```python
from build123d import *

# Parameters (mm, degrees)
SKETCH1_W           = 145
SKETCH1_H           = 25
BOSS_EXTRUDE1_DEPTH = 10
SKETCH2_W           = 17.5
SKETCH2_H           = 32
BOSS_EXTRUDE2_DEPTH = 10
SKETCH4_W           = 73.5
SKETCH4_H           = 32
BOSS_EXTRUDE3_DEPTH = 10
SKETCH8_R           = 2.25
CUT_EXTRUDE5_DEPTH  = 193.888568868
SKETCH9_W           = 7.3
SKETCH9_H           = 4
CUT_EXTRUDE6_DEPTH  = 10
CUT_EXTRUDE7_REACH  = 195.92
SKETCH10_R          = 3.65
SKETCH11_R          = 12.75
CUT_EXTRUDE8_DEPTH  = 7
CUT_EXTRUDE11_REACH = 196.098
SKETCH14_R          = 1.65
CHAMFER1_SIZE       = 1.5
CHAMFER1_SIZE2      = 0.866025404
FILLET1_R           = 15
SKETCH15_R          = 2.25
CUT_EXTRUDE12_DEPTH = 195.692064553
CUT_EXTRUDE13_DEPTH = 4


with BuildPart() as part:
    # Sketch1 → Boss-Extrude1 (new body)
    with BuildSketch(Plane(origin=(0, 0, 0), x_dir=(1, 0, 0), z_dir=(0, 1, 0))):
        with Locations((72.5, 12.5)):
            Rectangle(SKETCH1_W, SKETCH1_H)
    extrude(amount=BOSS_EXTRUDE1_DEPTH)

    # Sketch2 → Boss-Extrude2 (add)
    with BuildSketch(Plane(origin=(0, 10, 0), x_dir=(1, 0, 0), z_dir=(0, 1, 0))):
        with Locations((153.75, 16)):
            Rectangle(SKETCH2_W, SKETCH2_H)
    extrude(amount=-BOSS_EXTRUDE2_DEPTH)

    # Sketch4 → Boss-Extrude3 (add)
    with BuildSketch(Plane.XZ):
        with Locations((154.25, -16)):
            Rectangle(SKETCH4_W, SKETCH4_H)
    extrude(amount=BOSS_EXTRUDE3_DEPTH)

    # Sketch8 → Cut-Extrude5 (cut, through all)
    with BuildSketch(Plane(origin=(0, 0, -25), x_dir=(-1, 0, 0), z_dir=(0, 0, -1))):
        with Locations((-137, 5)):
            Circle(SKETCH8_R)
        with Locations((-101, 5)):
            Circle(SKETCH8_R)
        with Locations(Location((-44, 5, 0), (0, 0, 180))):
            Circle(SKETCH8_R)
        with Locations(Location((-8, 5, 0), (0, 0, 180))):
            Circle(SKETCH8_R)
    extrude(amount=-CUT_EXTRUDE5_DEPTH, mode=Mode.SUBTRACT)

    # Sketch9 → Cut-Extrude6 (cut)
    with BuildSketch(Plane(origin=(0, 10, 0), x_dir=(1, 0, 0), z_dir=(0, 1, 0))):
        with Locations((137, 20)):
            Rectangle(SKETCH9_W, SKETCH9_H)
        with Locations((137, 5)):
            Rectangle(SKETCH9_W, SKETCH9_H)
        with Locations((101, 5)):
            Rectangle(SKETCH9_W, SKETCH9_H)
        with Locations((101, 20)):
            Rectangle(SKETCH9_W, SKETCH9_H)
        with Locations((8, 20)):
            Rectangle(SKETCH9_W, SKETCH9_H)
        with Locations((44, 20)):
            Rectangle(SKETCH9_W, SKETCH9_H)
        with Locations((44, 5)):
            Rectangle(SKETCH9_W, SKETCH9_H)
        with Locations((8, 5)):
            Rectangle(SKETCH9_W, SKETCH9_H)
    extrude(amount=-CUT_EXTRUDE6_DEPTH, mode=Mode.SUBTRACT)

    # Sketch10 → Cut-Extrude7 (cut, up to next)
    with BuildSketch(Plane(origin=(0, 0, 0), x_dir=(1, 0, 0), z_dir=(0, 1, 0)), mode=Mode.PRIVATE) as cut_extrude7_sk1:
        with Locations(Location((176, 16, 0), (0, 0, 270))):
            Circle(SKETCH10_R)
    cut_extrude7_tool1 = extrude(cut_extrude7_sk1.sketch, amount=-CUT_EXTRUDE7_REACH, mode=Mode.PRIVATE) & part.part
    add(cut_extrude7_tool1.solids().sort_by_distance((176, 0, -16))[0], mode=Mode.SUBTRACT)

    # Sketch11 → Cut-Extrude8 (cut)
    with BuildSketch(Plane.XZ.offset(10)):
        with Locations(Location((176, -16, 0), (0, 0, 270))):
            Circle(SKETCH11_R)
    extrude(amount=-CUT_EXTRUDE8_DEPTH, mode=Mode.SUBTRACT)

    # Sketch14 → Cut-Extrude11 (cut, up to next)
    with BuildSketch(Plane.XZ.offset(3), mode=Mode.PRIVATE) as cut_extrude11_sk1:
        with Locations(Location((176, -7.5, 0), (0, 0, 270))):
            Circle(SKETCH14_R)
    cut_extrude11_tool1 = extrude(cut_extrude11_sk1.sketch, amount=-CUT_EXTRUDE11_REACH, mode=Mode.PRIVATE) & part.part
    # Sketch14 → Cut-Extrude11 (cut, up to next)
    with BuildSketch(Plane.XZ.offset(3), mode=Mode.PRIVATE) as cut_extrude11_sk2:
        with Locations(Location((176, -24.5, 0), (0, 0, 270))):
            Circle(SKETCH14_R)
    cut_extrude11_tool2 = extrude(cut_extrude11_sk2.sketch, amount=-CUT_EXTRUDE11_REACH, mode=Mode.PRIVATE) & part.part
    add(cut_extrude11_tool1.solids().sort_by_distance((176, -3, -7.5))[0], mode=Mode.SUBTRACT)
    add(cut_extrude11_tool2.solids().sort_by_distance((176, -3, -24.5))[0], mode=Mode.SUBTRACT)

    # Chamfer1
    chamfer1_edges = [part.edges().sort_by_distance(p)[0] for p in [
        (176, 0, -5.85),
        (176, 0, -22.85),
    ]]
    chamfer1_side = [part.faces().sort_by_distance(p)[0] for p in [
        (162.928514877, 0, -16),
    ]]
    chamfer(chamfer1_edges, length=CHAMFER1_SIZE, length2=CHAMFER1_SIZE2, reference=chamfer1_side[0])

    # Fillet1
    fillet1_edges = [part.edges().sort_by_distance(p)[0] for p in [
        (162.5, 5, -32),
        (162.5, 5, 0),
        (191, -5, -32),
        (191, -5, 0),
    ]]
    fillet(fillet1_edges, radius=FILLET1_R)

    # Sketch15 → Cut-Extrude12 (cut, through all)
    with BuildSketch(Plane(origin=(0, 10, 0), x_dir=(1, 0, 0), z_dir=(0, 1, 0))):
        with Locations(Location((57.5, 12.5, 0), (0, 0, 270))):
            Circle(SKETCH15_R)
        with Locations(Location((87.5, 12.5, 0), (0, 0, 270))):
            Circle(SKETCH15_R)
    extrude(amount=-CUT_EXTRUDE12_DEPTH, mode=Mode.SUBTRACT)

    # Sketch16 → Cut-Extrude13 (cut)
    with BuildSketch(Plane(origin=(0, 10, 0), x_dir=(1, 0, 0), z_dir=(0, 1, 0))):
        Polygon((91.714656965, 12.5), (89.607328483, 16.15), (85.392671517, 16.15), (83.285343035, 12.5), (85.392671517, 8.85), (89.607328483, 8.85), align=None)
        Polygon((61.714656965, 12.5), (59.607328483, 16.15), (55.392671517, 16.15), (53.285343035, 12.5), (55.392671517, 8.85), (59.607328483, 8.85), align=None)
    extrude(amount=-CUT_EXTRUDE13_DEPTH, mode=Mode.SUBTRACT)


solid = part.part
```
Design review of the part built by this model. Coordinates are the model's own, in mm. A direction names the side the tool comes from. Coordinates: 2 decimals unless noted, no trailing zeros. Write each loop counter-clockwise with the first axis right and the second up, starting at its lowest first coordinate (ties: lowest second). Pieces come first, ordered by that corner, then holes.
1) Add section B-B (y = -8). Write out the cut boundary in (x, z), plus the area to 3 significant figures.
2) Add section C-C (x = 142.5). Write out the cut boundary in (y, z).
3) Add section D-D (x = 32). Write out the cut boundary in (y, z), plus the area to 3 significant figures.
4) Mouldability with a two-part tool opening along X and no side actions: class faces 4 (the flat face through (133.35, 5, -5)), 5 (the flat face through (131, 0, -28)), 6 (the flat face through (140.65, 5, -20)) as +X half, -X half, draft (parallel to the pull), parting line (faces both ways), or undercut.
5) Add section A-A (x = 87.5). Write out the cut boundary in (y, z).
6) To check wall thickness, follow L1, parallel to Z at x = 46, y = 7.5; L2, parallel to X at y = -1.75, z = -16.5; L3, parallel to Y at x = 137, z = -15.5. State the ranges of each line that lie inside material, in increasing order.
7) Machinability: for faces 1 (the flat face through (60.646, 8.028, -10.649)), 2 (the flat face through (104.65, 5, -5)), 3 (the cylindrical face through (98.92, 4.14, -1.52)), which of the approach directions +Z, -Z, +X, -X, +Y, -Y give a long, thin tool a straight path to every point of the face, cutting with its end or side? Answer none if there is none.
8) Insertion check: pin 1 (3 mm diameter, centred on y = 7, z = -21, fed in from +X); pin 2 (3.5 mm diameter, centred on x = 8, y = 5, fed in from -Z); pin 3 (7.5 mm diameter, centred on x = 63, z = -8.5, fed in from -Y); pin 4 (3 mm diameter, centred on y = 6, z = -4, fed in from +X). Each pin has a flat end and moves straight along its axis. Give the tip position at first contact, or say it passes through.
Check result:
1. outline: (117.5, -32) - (176, -32) arc R15 ccw to (191, -17) - (191, -15) arc R15 ccw to (176, 0) - (117.5, 0) - close; hole circle Ø25.5 at (176, -16)
1. area: 1,740 mm2
2. outline: (-10, -32) - (0, -32) - (0, -25) - (10, -25) - (10, 0) - (-10, 0) - close
3. outline: (0, -25) - (10, -25) - (10, 0) - (0, 0) - close
3. area: 250 mm2
4. face 4: undercut
4. face 5: draft
4. face 6: undercut
5. outline: (0, -25) - (10, -25) - (10, -16.15) - (6, -16.15) - (6, -14.75) - (0, -14.75) - close; (0, -10.25) - (6, -10.25) - (6, -8.85) - (10, -8.85) - (10, 0) - (0, 0) - close
6. L1: z = -25 to -22, -18 to -7, -3 to 0
6. L2: x = 117.5 to 172.38, 179.62 to 191
6. L3: y = -10 to 2.75, 7.25 to 10
7. face 1: +Y
7. face 2: +Y, -Y
7. face 3: +Z, -Z
8. pin 1: stops at x = 162.29
8. pin 2: passes through
8. pin 3: stops at y = 0
8. pin 4: stops at x = 159.11
